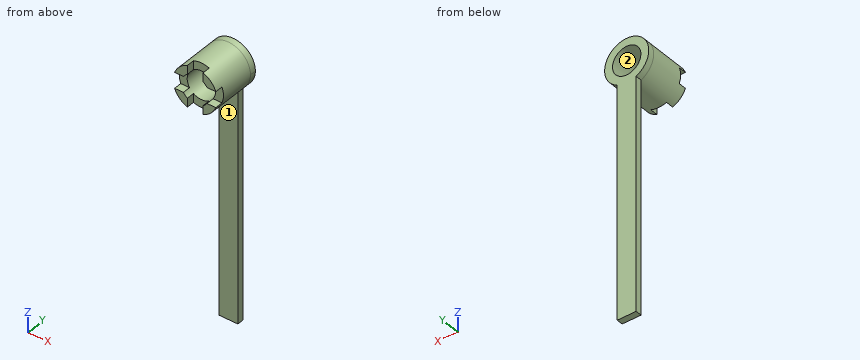
```python
from build123d import *

# Parameters (mm, degrees)
BOSS_EXTRUDE1_DEPTH = 2.54
BOSS_EXTRUDE2_START = 17.145
SKETCH3_R           = 8.89
SKETCH3_R_2         = 5.715
BOSS_EXTRUDE2_DEPTH = 17.145
CUT_EXTRUDE1_DEPTH  = 3.175


with BuildPart() as part:
    # Sketch2 → Boss-Extrude1 (new body)
    with BuildSketch(Plane(origin=(0, 0, 0), x_dir=(1, 0, 0), z_dir=(0, 1, 0))):
        with BuildLine():
            Line((3.81, 8.032185257), (3.81, 101.6))
            Line((3.81, 101.6), (-3.81, 101.6))
            Line((-3.81, 101.6), (-3.81, 8.032185257))
            ThreePointArc((-3.81, 8.032185257), (0, 8.89), (3.81, 8.032185257))
        make_face()
        with BuildLine():
            ThreePointArc((8.89, 0), (7.513421325, 4.751904881), (3.81, 8.032185257))
            Line((3.81, 8.032185257), (3.81, 4.259709497))
            ThreePointArc((3.81, 4.259709497), (5.21705736, 2.33313898), (5.715, 0))
            ThreePointArc((5.715, 0), (-2.33313898, -5.21705736), (-3.81, 4.259709497))
            Line((-3.81, 4.259709497), (-3.81, 8.032185257))
            ThreePointArc((-3.81, 8.032185257), (-4.751904881, -7.513421325), (8.89, 0))
        make_face()
        with BuildLine():
            Line((3.81, 4.259709497), (3.81, 8.032185257))
            ThreePointArc((3.81, 8.032185257), (0, 8.89), (-3.81, 8.032185257))
            Line((-3.81, 8.032185257), (-3.81, 4.259709497))
            ThreePointArc((-3.81, 4.259709497), (0, 5.715), (3.81, 4.259709497))
        make_face()
    extrude(amount=BOSS_EXTRUDE1_DEPTH)

    # Sketch3 → Boss-Extrude2 (add)
    with BuildSketch(Plane.XZ.offset(BOSS_EXTRUDE2_START)):
        with Locations(Location((0, 0, 0), (0, 0, 270))):
            Circle(SKETCH3_R)
        with Locations(Location((0, 0, 0), (0, 0, 270))):
            Circle(SKETCH3_R_2, mode=Mode.SUBTRACT)
    extrude(amount=-BOSS_EXTRUDE2_DEPTH)

    # Sketch4 → Cut-Extrude1 (cut)
    with BuildSketch(Plane.XZ.offset(17.145)):
        with BuildLine():
            Line((-4.751904881, 3.175), (-8.303702487, 3.175))
            ThreePointArc((-8.303702487, 3.175), (-8.89, 0), (-8.303702487, -3.175))
            Line((-8.303702487, -3.175), (-4.751904881, -3.175))
            ThreePointArc((-4.751904881, -3.175), (-5.715, 0), (-4.751904881, 3.175))
        make_face()
        with BuildLine():
            ThreePointArc((8.89, 0), (8.742196953, 1.614339631), (8.303702487, 3.175))
            Line((8.303702487, 3.175), (4.751904881, 3.175))
            ThreePointArc((4.751904881, 3.175), (5.468928661, 1.658928661), (5.715, 0))
            ThreePointArc((5.715, 0), (5.468928661, -1.658928661), (4.751904881, -3.175))
            Line((4.751904881, -3.175), (8.303702487, -3.175))
            ThreePointArc((8.303702487, -3.175), (8.742196953, -1.614339631), (8.89, 0))
        make_face()
        with BuildLine():
            ThreePointArc((3.175, 8.303702487), (0, 8.89), (-3.175, 8.303702487))
            Line((-3.175, 8.303702487), (-3.175, 4.751904881))
            ThreePointArc((-3.175, 4.751904881), (0, 5.715), (3.175, 4.751904881))
            Line((3.175, 4.751904881), (3.175, 8.303702487))
        make_face()
        with BuildLine():
            Line((-3.175, -4.751904881), (-3.175, -8.303702487))
            ThreePointArc((-3.175, -8.303702487), (0, -8.89), (3.175, -8.303702487))
            Line((3.175, -8.303702487), (3.175, -4.751904881))
            ThreePointArc((3.175, -4.751904881), (0, -5.715), (-3.175, -4.751904881))
        make_face()
    extrude(amount=-CUT_EXTRUDE1_DEPTH, mode=Mode.SUBTRACT)


solid = part.part
```
Model file for the job. Use its own axes, mm. Face numbers are marked on the shaded views. Round coordinates to 2 decimals unless told otherwise and drop trailing zeros. Write each loop counter-clockwise with the first axis right and the second up, starting at its lowest first coordinate (ties: lowest second). Pieces come first, ordered by that corner, then holes. Notation, with made-up numbers: M 20,-7.5 L 60,-7.5 A18 ccw 60,10.5 Z; hole C -18,0 d2. An arc over 180 degrees is marked long. Put each result on its own line as item: value.
Item 1: Flat gauge pins, fed straight in: P1, Ø8.5, axis at x = -0.5, z = -61.5, coming from the -Y side; P2, Ø5, axis at x = 5.5, y = -11, coming from the +Z side; P3, Ø1.3, axis at y = 1.5, z = -39.5, coming from the -X side. Where does each tip first touch, or does it go through?
Responses:
P1: y = 0
P2: z = 8.37
P3: x = -3.81
Item 2: Cut at C-C (z = -67.5). List the corners of the cut face in (x, y), and give its area (3 significant figures).
Responses:
outline: M -3.81,0 L 3.81,0 L 3.81,2.54 L -3.81,2.54 Z
area: 19.4 mm²
Item 3: Mould opens along Z. For the marked faces 1 and 2 say: +Z half, -Z half, draft (parallel to the pull), parting line (faces both ways), or undercut.
Responses:
face 1: draft
face 2: undercut
Item 4: Cut at A-A (x = 2). List the corners of the cut face in (y, z), and give its area (3 significant figures).
Responses:
outline: M -13.97,-8.66 L 0,-8.66 L 0,-101.6 L 2.54,-101.6 L 2.54,-5.35 L -13.97,-5.35 Z; M -13.97,5.35 L 2.54,5.35 L 2.54,8.66 L -13.97,8.66 Z
area: 345 mm²
Item 5: Probe L1, parallel to X at y = -1.5, z = 0 (3 decimals); L2, parallel to X at y = 1.25, z = -22. List the from-to ranges inside material, lowest first. Write a range as from..to.
Responses:
L1: -8.89..-5.715, 5.715..8.89
L2: -3.81..3.81
Item 6: Cut at B-B (y = -12). List the corners of the cut face in (x, z) (3 decimals), and give its area (3 significant figures).
Responses:
outline: C 0,0 d17.78; hole C 0,0 d11.43
area: 146 mm²
